Source: CAD feature listing. Evaluate the final solid. Frame: model axes, mm. Face numbers are marked on the shaded views. A direction names the side the tool comes from. Give positions to 0.01 mm unless a question says otherwise; leave off trailing zeros. Order: outer loops, then holes, each group sorted by start corner. A loop starts at its lowest first (then second) coordinate and runs counter-clockwise, first axis right, second up.
1) Section D-D, the plane z = -5.5. Return loops of the section in (x, y), plus the area to 3 significant figures.
2) Section C-C, the plane y = 1.25. Return loops of the section in (x, z), plus the area to 3 significant figures.
3) First-contact query: P1, Ø1.8, axis at x = 0, z = 4.76, coming from the +Y side; P2, Ø2.5, axis at x = 0, z = -4.76, coming from the -Y side; P3, Ø0.6, axis at x = 0.5, y = 0.5, coming from the +Z side. Flat tips, straight axial feed; report the tip coordinate or a pass-through.
4) Section A-A, the plane z = 0. Return loops of the section in (x, y), plus the area to 4 significant figures.
5) Section B-B, the plane x = 0. Return loops of the section in (y, z).
6) Draft query along X for the marked faces 4, 5, 6 and 7. Return one class per face: released by +X, released by -X, zero draft, split by the parting line, or undercut.
7) Material intervals for line 1 (X direction, y = 1.8, z = 0); line 2 (Z direction, x = 0.75, y = 1.3); line 3 (Y direction, x = 5, z = -0.5), sorted ascending.
8) Access query for the marked faces 1, 2 and 3. Directions: +Z, -Z, +X, -X, +Y, -Y. A direction counts if a zero-diameter tool reaches every point of the face in a straight line with its end or side. Return the directions, or none.
```python
from build123d import *

# Parameters (mm, degrees)
SKETCH2_R           = 6.35
SKETCH2_W           = 3.175
SKETCH2_H           = 3.175
BOSS_EXTRUDE1_DEPTH = 2
SKETCH3_R           = 1
CUT_EXTRUDE1_DEPTH  = 1
CIRPATTERN1_COUNT   = 4


with BuildPart() as part:
    # Sketch2 → Boss-Extrude1 (new body)
    with BuildSketch(Plane(origin=(0, 0, 0), x_dir=(1, 0, 0), z_dir=(0, 1, 0))):
        with Locations(Location((0, 0, 0), (0, 0, 270))):
            Circle(SKETCH2_R)
        Rectangle(SKETCH2_W, SKETCH2_H, mode=Mode.SUBTRACT)
    extrude(amount=BOSS_EXTRUDE1_DEPTH)

    # Sketch3 → Cut-Extrude1 (cut)
    with BuildSketch(Plane(origin=(0, 2, 0), x_dir=(1, 0, 0), z_dir=(0, 1, 0))):
        with Locations(Location((-4.7625, 0, 0), (0, 0, 270))):
            Circle(SKETCH3_R)
    cut_extrude1 = extrude(amount=-CUT_EXTRUDE1_DEPTH, mode=Mode.SUBTRACT)

    # CirPattern1: Cut-Extrude1 ×4 about axis
    cirpattern1_axis = Axis((0, 0, 0), (0, 1, 0))
    for i in range(1, CIRPATTERN1_COUNT):
        add(cut_extrude1.rotate(cirpattern1_axis, i * 360 / CIRPATTERN1_COUNT), mode=Mode.SUBTRACT)


solid = part.part
```
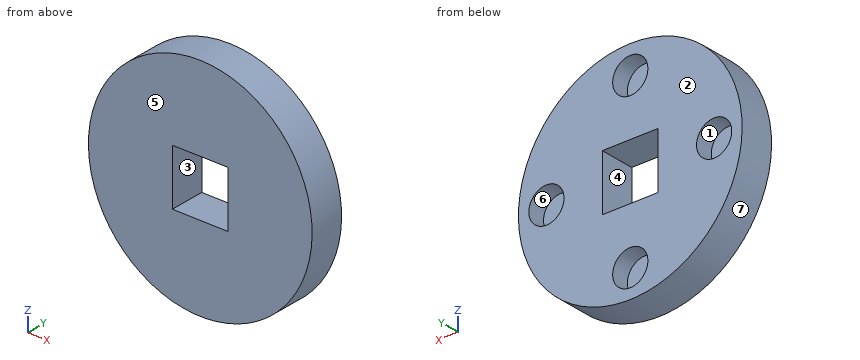
From the geometry:
1. outline: (-3.17, 0) - (3.17, 0) - (3.17, 2) - (0.68, 2) - (0.68, 1) - (-0.68, 1) - (-0.68, 2) - (-3.17, 2) - close
1. area: 11.3 mm2
2. outline: circle Ø12.7 at (0, 0); hole circle Ø2 at (-4.76, 0); hole (-1.59, -1.59) - (1.59, -1.59) - (1.59, 1.59) - (-1.59, 1.59) - close; hole circle Ø2 at (0, -4.76); hole circle Ø2 at (0, 4.76); hole circle Ø2 at (4.76, 0)
2. area: 104 mm2
3. P1: stops at y = 1
3. P2: stops at y = 0
3. P3: stops at z = 6.35
4. outline: (-6.35, 0) - (-1.59, 0) - (-1.59, 2) - (-3.76, 2) - (-3.76, 1) - (-5.76, 1) - (-5.76, 2) - (-6.35, 2) - close; (1.59, 0) - (6.35, 0) - (6.35, 2) - (5.76, 2) - (5.76, 1) - (3.76, 1) - (3.76, 2) - (1.59, 2) - close
4. area: 15.05 mm2
5. outline: (0, -6.35) - (2, -6.35) - (2, -5.76) - (1, -5.76) - (1, -3.76) - (2, -3.76) - (2, -1.59) - (0, -1.59) - close; (0, 1.59) - (2, 1.59) - (2, 3.76) - (1, 3.76) - (1, 5.76) - (2, 5.76) - (2, 6.35) - (0, 6.35) - close
6. face 4: undercut
6. face 5: zero draft
6. face 6: undercut
6. face 7: split by the parting line
7. line 1: x = -6.35 to -5.76, -3.76 to -1.59, 1.59 to 3.76, 5.76 to 6.35
7. line 2: z = -6.31 to -5.42, -4.1 to -1.59, 1.59 to 4.1, 5.42 to 6.31
7. line 3: y = 0 to 1
8. face 1: +Y
8. face 2: +Z, -Z, +X, -X, +Y
8. face 3: +Y, -Y
